from build123d import *

# Parameters (mm, degrees)
PAD_DEPTH    = 120
SKETCH001_R  = 1.75
PAD001_DEPTH = 3
FILLET_R     = 3


with BuildPart() as part:
    # Sketch → Pad (new body)
    with BuildSketch(Plane.XY):
        Polygon((0, 0), (74, 0), (74, 11), (72, 11), (72, 10), (73, 10), (73, 9), (72, 9), (72, 2), (57.5, 2), (57.5, 9), (56.5, 9), (56.5, 10), (57.5, 10), (57.5, 11), (53.5, 11), (53.5, 10), (54.5, 10), (54.5, 9), (53.5, 9), (53.5, 2), (39, 2), (39, 9), (38, 9), (38, 10), (39, 10), (39, 11), (35, 11), (35, 10), (36, 10), (36, 9), (35, 9), (35, 2), (20.5, 2), (20.5, 9), (19.5, 9), (19.5, 10), (20.5, 10), (20.5, 11), (16.5, 11), (16.5, 10), (17.5, 10), (17.5, 9), (16.5, 9), (16.5, 2), (2, 2), (2, 9), (1, 9), (1, 10), (2, 10), (2, 11), (0, 11), align=None)
    extrude(amount=PAD_DEPTH)

    # Sketch001 → Pad001 (join)
    with BuildSketch(Plane.XZ):
        Polygon((0, 4.994447), (-13, 12.5), (-13, 17.5), (0, 25.005553), align=None)
        with Locations((-8, 15)):
            Circle(SKETCH001_R, mode=Mode.SUBTRACT)
        Polygon((0, 65.005553), (-13, 72.5), (-13, 77.5), (0, 84.994447), align=None)
        with Locations((-8, 75)):
            Circle(SKETCH001_R, mode=Mode.SUBTRACT)
        Polygon((74, 35.494447), (87, 43), (87, 48), (74, 55.505553), align=None)
        with Locations((82, 45)):
            Circle(SKETCH001_R, mode=Mode.SUBTRACT)
        Polygon((74, 94.994447), (87, 102.5), (87, 107.5), (74, 115.005553), align=None)
        with Locations((82, 105)):
            Circle(SKETCH001_R, mode=Mode.SUBTRACT)
    extrude(amount=-PAD001_DEPTH)

    # Fillet
    fillet_edges = [part.edges().sort_by_distance(p)[0] for p in [
        (39, 2, 60),
        (57.5, 2, 60),
        (72, 2, 60),
        (53.5, 2, 60),
        (2, 2, 60),
        (20.5, 2, 60),
        (16.5, 2, 60),
        (35, 2, 60),
    ]]
    fillet(fillet_edges, radius=FILLET_R)


solid = part.part
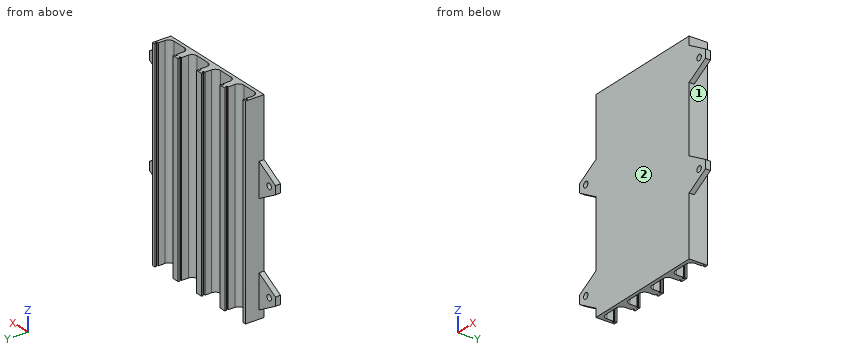
The model under review builds one solid part; all positions refer to its coordinate system, in mm. Face numbers are marked on the shaded views. A direction names the side the tool comes from. Round coordinates to 2 decimals unless told otherwise and drop trailing zeros. Write each loop counter-clockwise with the first axis right and the second up, starting at its lowest first coordinate (ties: lowest second). Pieces come first, ordered by that corner, then holes. Notation, with made-up numbers: M 66.5,26 L 95.5,26 A24 ccw 95.5,40 Z; hole C 41,31 d7. An arc over 180 degrees is marked long. Answer as CSV lines item,"result". Start each with the question number.
Q1. Clearance check with flat-ended pins moving along their axes: P1, Ø6.5, axis at x = 79, z = 50, coming from the +Y side; P2, Ø5.5, axis at y = 8, z = 33.5, coming from the +X side; P3, Ø7, axis at x = 48.5, z = 65, coming from the +Y side; P4, Ø3, axis at x = 82, z = 105, coming from the -Y side. State where each tip first meets the part, or that it passes through.
Q2. Wall thickness on line 1 along X through (y, z) = (7.25, 63); line 2 along X through (y, z) = (1.8, 75); line 3 along Z through (x, y) = (82, 1): over which ranges is each line inside the solid? List them lowest first.
Q3. Consider section A-A, the plane y = 7.5. Give the boundary of the cut face in (x, z).
Q4. Tool access review of the marked faces 1 and 2: name each direction out of +Z, -Z, +X, -X, +Y, -Y from which nothing blocks a thin tool from reaching the whole face with its end or side.
Q5. Consider section C-C, the plane x = 10. Give the boundary of the cut face in (y, z).
Q6. Consider section B-B, the plane x = -8. Give the boundary of the cut face in (y, z).
Result set:
1,P1,"stops at y = 3"
1,P2,"stops at x = 74"
1,P3,"stops at y = 2.4"
1,P4,"passes through"
2,line 1,"x = 0 to 2, 16.5 to 20.5, 35 to 39, 53.5 to 57.5, 72 to 74"
2,line 2,"x = -13 to -9.75, -6.25 to 74"
2,line 3,"z = 40.11 to 43.25, 46.75 to 50.89, 99.61 to 103.25, 106.75 to 110.39"
3,outline,"M 0,0 L 2,0 L 2,120 L 0,120 Z; M 16.5,0 L 20.5,0 L 20.5,120 L 16.5,120 Z; M 35,0 L 39,0 L 39,120 L 35,120 Z; M 53.5,0 L 57.5,0 L 57.5,120 L 53.5,120 Z; M 72,0 L 74,0 L 74,120 L 72,120 Z"
4,face 1,"+X, +Y"
4,face 2,"+Z, -Z, +X, -X, -Y"
5,outline,"M 0,0 L 2,0 L 2,120 L 0,120 Z"
6,outline,"M 0,9.61 L 3,9.61 L 3,13.25 L 0,13.25 Z; M 0,16.75 L 3,16.75 L 3,20.39 L 0,20.39 Z; M 0,69.62 L 3,69.62 L 3,73.25 L 0,73.25 Z; M 0,76.75 L 3,76.75 L 3,80.38 L 0,80.38 Z"
